Geometry: final body of the model. Coordinates: model frame, mm. A direction names the side the tool comes from. Give positions to 0.01 mm unless a question says otherwise; leave off trailing zeros. Loops run counter-clockwise (first coordinate to the right, second up) from the corner with the lowest first, then second, coordinate; pieces in that order, holes last. Notation, with made-up numbers: (-12, 57.5) - (26, 57.5) arc R28 cw to (26, 86.5) - close; hole circle Ø2 at (12, 58). An arc over 180 degrees is marked (long way). Use one line per item in the form item = value.
```python
from build123d import *

# Parameters (mm, degrees)
BOSS_EXTRUDE1_DEPTH = 9
SKETCH2_R           = 1.5
BOSS_EXTRUDE2_DEPTH = 7
SKETCH3_W           = 3.75
SKETCH3_H           = 2.16506351
BOSS_EXTRUDE3_DEPTH = 9
SKETCH4_W           = 0.75
SKETCH4_H           = 4
CUT_EXTRUDE1_DEPTH  = 19.650150804
SKETCH5_R           = 1.5
CUT_EXTRUDE2_DEPTH  = 19.460684576


with BuildPart() as part:
    # Sketch1 → Boss-Extrude1 (new body)
    with BuildSketch(Plane(origin=(0, 0, 0), x_dir=(1, 0, 0), z_dir=(0, 1, 0))):
        Polygon((2.5, 0), (1.25, 2.165063509), (-1.25, 2.165063509), (-2.5, 0), (-1.25, -2.165063509), (1.25, -2.165063509), align=None)
    extrude(amount=BOSS_EXTRUDE1_DEPTH)

    # Sketch2 → Boss-Extrude2 (add)
    with BuildSketch(Plane.XZ):
        with Locations(Location((0, 0, 0), (0, 0, 270))):
            Circle(SKETCH2_R)
    extrude(amount=BOSS_EXTRUDE2_DEPTH)

    # Sketch3 → Boss-Extrude3 (add)
    with BuildSketch(Plane(origin=(0, 9, 0), x_dir=(1, 0, 0), z_dir=(0, 1, 0))):
        Rectangle(SKETCH3_W, SKETCH3_H)
    extrude(amount=BOSS_EXTRUDE3_DEPTH)

    # Sketch4 → Cut-Extrude1 (cut, through all)
    with BuildSketch(Plane.ZY.offset(1.875)):
        with Locations((-0.707531755, 11)):
            Rectangle(SKETCH4_W, SKETCH4_H)
        with Locations((0.707531755, 11)):
            Rectangle(SKETCH4_W, SKETCH4_H)
    extrude(amount=-CUT_EXTRUDE1_DEPTH, mode=Mode.SUBTRACT)

    # Sketch5 → Cut-Extrude2 (cut, through all)
    with BuildSketch(Plane(origin=(0, 0, -1.082531755), x_dir=(-1, 0, 0), z_dir=(0, 0, -1))):
        with Locations((0, 16.25)):
            Circle(SKETCH5_R)
        with BuildLine():
            ThreePointArc((-1.75, 16.25), (-1.237436867, 17.487436868), (2e-09, 18))
            Line((2e-09, 18), (-1.875, 18))
            Line((-1.875, 18), (-1.875, 13))
            Line((-1.875, 13), (-1.75, 16.25))
        make_face()
        with BuildLine():
            ThreePointArc((2e-09, 18), (1.237436868, 17.487436867), (1.75, 16.25))
            Line((1.75, 16.25), (1.875, 13))
            Line((1.875, 13), (1.875, 18))
            Line((1.875, 18), (2e-09, 18))
        make_face()
    extrude(amount=-CUT_EXTRUDE2_DEPTH, mode=Mode.SUBTRACT)

    # Mirror1: part across plane


with BuildPart() as part_1:
    add(part.part)
    add(part.part.mirror(Plane(origin=(0, -7, 0), x_dir=(0, 0, 1), z_dir=(0, -1, 0))))


solid = part_1.part
```
(1) Cut plane A-A (y = -10). Return the cut outline in (x, z), plus the area to 3 significant figures.
Solution:
outline = circle Ø3 at (0, 0)
area = 7.07 mm2
(2) Pin query (flat end, axial travel): P1, Ø1.9, axis at x = 0, y = -28.5, coming from the +Z side; P2, Ø0.8, axis at x = -0.5, z = -0.5, coming from the -Y side; P3, Ø1.1, axis at x = 0.5, y = 15.5, coming from the +Z side; P4, Ø0.7, axis at y = -24.5, z = 0, coming from the -X side (3 decimals). Return the tip coordinate at first contact, or that it passes through.
Solution:
P1 = 1.08
P2 = -32
P3 = through
P4 = -1.875
(3) Material intervals for L1, parallel to Y at x = 0, z = 0.3; L2, parallel to Y at x = 1.15, z = 1.35; L3, parallel to Y at x = -0.8, z = -0.3, sorted ascending. Write a range as from..to.
Solution:
L1 = -32..-31.75, -28.75..14.75, 17.75..18
L2 = -23..-14, 0..9
L3 = -31.81..-31.52, -28.98..14.98, 17.52..17.81
(4) Access query for faces 1 (the face through (0, 11, -0.333)), 2 (the face through (0, 14, -1.083)), 3 (the face through (0, 11, 0.333)). Directions: +Z, -Z, +X, -X, +Y, -Y. A direction counts if a zero-diameter tool reaches every point of the face in a straight line with its end or side. Return the directions, or none.
Solution:
face_1 = -Z, +X, -X
face_2 = -Z, +X, -X, +Y
face_3 = +Z, +X, -X
(5) Pull-direction query (X, two-part tool) for faces 4 (the face through (1.11, 17.26, -0.02)), 5 (the face through (0, -25, -0.333)), 6 (the face through (-1.88, -18.44, 1.07)); classes: released by +X, released by -X, zero draft, split by the parting line, or undercut.
Solution:
face_4 = undercut
face_5 = zero draft
face_6 = released by -X
